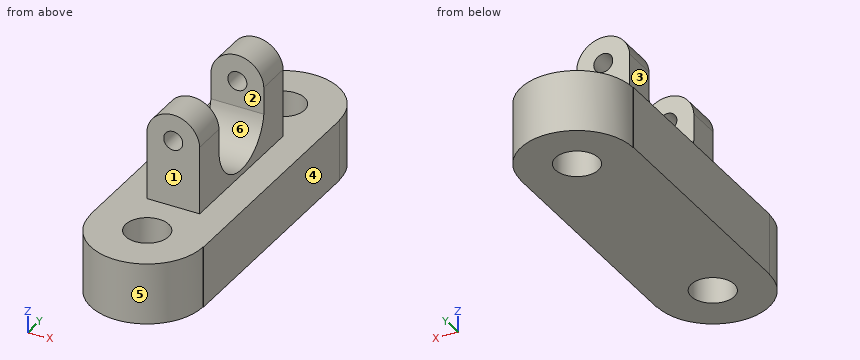
from build123d import *

# Parameters (mm, degrees)
F0_R     = 13.378709
F1_DEPTH = 38.1
F2_W     = 32.905034
F2_H     = 93.086616
F3_DEPTH = 63.5
F4_R     = 5.910106
F5_DEPTH = 157.258617
F6_W     = 49.855356
F6_H     = 31.583474
F7_DEPTH = 51.616201


with BuildPart() as f1:
    # F0 (on Top) → F1 (new body)
    with BuildSketch(Plane.XY):
        with BuildLine():
            Line((-34.876153, 75.838156), (-35.162684, 75.838156))
            Line((-35.162684, 75.838156), (-35.162684, -75.838156))
            Line((-35.162684, -75.838156), (-34.876156, -75.838156))
            ThreePointArc((-34.876156, -75.838156), (-3e-06, -110.714309), (34.87615, -75.838156))
            Line((34.87615, -75.838156), (35.162684, -75.838156))
            Line((35.162684, -75.838156), (35.162684, 75.838156))
            Line((35.162684, 75.838156), (34.876153, 75.838156))
            ThreePointArc((34.876153, 75.838156), (0, 110.714309), (-34.876153, 75.838156))
        make_face()
        with Locations((-2e-06, -75.551689)):
            Circle(F0_R, mode=Mode.SUBTRACT)
        with Locations((0, 75.838156)):
            Circle(F0_R, mode=Mode.SUBTRACT)
    extrude(amount=F1_DEPTH)

    # F2 (on face) → F3 (join)
    with BuildSketch(Plane.XY.offset(38.1)):
        Rectangle(F2_W, F2_H)
    extrude(amount=F3_DEPTH)

    # F4 (on face) → F5 (cut, through all)
    with BuildSketch(Plane.XZ.offset(46.543308)):
        with BuildLine():
            ThreePointArc((-16.452517, 80.430904), (0, 96.095652), (16.452517, 80.430904))
            Line((16.452517, 80.430904), (16.452517, 101.6))
            Line((16.452517, 101.6), (-16.452517, 101.6))
            Line((-16.452517, 101.6), (-16.452517, 80.430904))
        make_face()
        with Locations((0, 79.623327)):
            Circle(F4_R)
    extrude(amount=-F5_DEPTH, mode=Mode.SUBTRACT)

    # F6 (on face) → F7 (cut, through all)
    with BuildSketch(Plane.YZ.offset(16.452517)):
        with BuildLine():
            Line((24.927678, 80.430904), (-24.927678, 80.430904))
            Line((-24.927678, 80.430904), (-24.927678, 63.47666))
            ThreePointArc((-24.927678, 63.47666), (0, 41.538121), (24.927678, 63.47666))
            Line((24.927678, 63.47666), (24.927678, 80.430904))
        make_face()
        with Locations((0, 96.222641)):
            Rectangle(F6_W, F6_H)
    extrude(amount=-F7_DEPTH, mode=Mode.SUBTRACT)


solid = f1.part
Read the model definition and answer for the solid it produces. Units are mm, in the model's axes. Face numbers are marked on the shaded views. A direction names the side the tool comes from. Round coordinates to 2 decimals unless told otherwise and drop trailing zeros. Loops run counter-clockwise (first coordinate to the right, second up) from the corner with the lowest first, then second, coordinate; pieces in that order, holes last.
Q1. Which of the six approach directions +Z, -Z, +X, -X, +Y, -Y give full straight-line access (tool end or side, diameter ignored) to the marked faces 1, 2 and 3?
Q2. Determine the mould class of the marked faces 4, 5 and 6 for opening direction Y: released by +Y, released by -Y, zero draft, split by the parting line, or undercut.
Q3. Each of these flat-tipped pins is pushed along its axis until it touches: pin 1 (1 mm diameter, centred on y = -36.5, z = 55.5, fed in from +X); pin 2 (3 mm diameter, centred on x = 15, z = 80, fed in from +Y); pin 3 (10.5 mm diameter, centred on x = 0, z = 79.62, fed in from +Y); pin 4 (3 mm diameter, centred on x = 1.5, z = 11.5, fed in from +Y). Where does it stop, or does it pass through?
Q4. Consider probe 1 along Y at (x, z) = (0, 20); probe 2 along Y at (x, z) = (-10, 92); probe 3 along Z at (x, y) = (0, -34.75). Determine where each line is inside the solid, lowest interval first.
Q5. Section D-D on z = 21.5 is taken. Write down the section's boundary in (x, y), and give its area (3 significant figures).
Q6. Section A-A on x = 0 is taken. Write down the section's boundary in (y, z), and give its area (3 significant figures).
Q7. Section C-C on x = -11 is taken. Write down the section's boundary in (y, z), and give its area (3 significant figures).
Q8. Section B-B on y = -84.5 is taken. Write down the section's boundary in (x, z), and give its area (3 significant figures).
Output:
1. face 1: +Z, +X, -X, -Y
1. face 2: +Z, +X, -X
1. face 3: +Z, -X, +Y, -Y
2. face 4: zero draft
2. face 5: released by -Y
2. face 6: undercut
3. pin 1: stops at x = 16.45
3. pin 2: stops at y = 46.54
3. pin 3: passes through
3. pin 4: stops at y = 110.71
4. probe 1: y = -110.71 to -88.93, -62.17 to 62.46, 89.22 to 110.71
4. probe 2: y = -46.54 to -24.93, 24.93 to 46.54
4. probe 3: z = 0 to 73.71, 85.53 to 96.1
5. outline: (-35.16, -75.84) - (-34.88, -75.84) arc R34.88 ccw to (34.88, -75.84) - (35.16, -75.84) - (35.16, 75.84) - (34.88, 75.84) arc R34.88 ccw to (-34.88, 75.84) - (-35.16, 75.84) - close; hole circle Ø26.76 at (0, -75.55); hole circle Ø26.76 at (0, 75.84)
5. area: 13,400 mm2
6. outline: (-110.71, 0) - (-88.93, 0) - (-88.93, 38.1) - (-110.71, 38.1) - close; (-62.17, 0) - (62.46, 0) - (62.46, 38.1) - (46.54, 38.1) - (46.54, 73.71) - (24.93, 73.71) - (24.93, 63.48) arc R25.13 cw to (-24.93, 63.48) - (-24.93, 73.71) - (-46.54, 73.71) - (-46.54, 38.1) - (-62.17, 38.1) - close; (-46.54, 85.53) - (-24.93, 85.53) - (-24.93, 96.1) - (-46.54, 96.1) - close; (24.93, 85.53) - (46.54, 85.53) - (46.54, 96.1) - (24.93, 96.1) - close; (89.22, 0) - (110.71, 0) - (110.71, 38.1) - (89.22, 38.1) - close
6. area: 8,830 mm2
7. outline: (-108.93, 0) - (-83.17, 0) - (-83.17, 38.1) - (-108.93, 38.1) - close; (-67.94, 0) - (68.22, 0) - (68.22, 38.1) - (46.54, 38.1) - (46.54, 91.88) - (24.93, 91.88) - (24.93, 63.48) arc R25.13 cw to (-24.93, 63.48) - (-24.93, 91.88) - (-46.54, 91.88) - (-46.54, 38.1) - (-67.94, 38.1) - close; (83.45, 0) - (108.93, 0) - (108.93, 38.1) - (83.45, 38.1) - close
7. area: 9,900 mm2
8. outline: (-33.78, 0) - (-9.95, 0) - (-9.95, 38.1) - (-33.78, 38.1) - close; (9.95, 0) - (33.78, 0) - (33.78, 38.1) - (9.95, 38.1) - close
8. area: 1,820 mm2
